Work out the finished part from the listing and answer in its coordinate system (mm). A direction names the side the tool comes from. Give positions to 0.01 mm unless a question says otherwise; leave off trailing zeros. Loops run counter-clockwise (first coordinate to the right, second up) from the corner with the lowest first, then second, coordinate; pieces in that order, holes last. Notation, with made-up numbers: (14, 46) - (19, 46) arc R12 ccw to (19, 61) - close; hole circle Ø7 at (-15.5, -2.5). An arc over 180 degrees is marked (long way). One line per question, with ' | ' between items.
from build123d import *

# Parameters (mm, degrees)
SKETCH1_R           = 4.3
SKETCH1_R_2         = 5.3
BOSS_EXTRUDE1_DEPTH = 3.3
SKETCH2_R           = 5.5
CUT_EXTRUDE1_DEPTH  = 93.907965213
FILLET1_R           = 2
SKETCH3_R           = 1.6
CUT_EXTRUDE2_DEPTH  = 93.907965213


with BuildPart() as part:
    # Sketch1 → Boss-Extrude1 (new body)
    with BuildSketch(Plane.ZY.offset(39)):
        with BuildLine():
            Line((61, 0), (21, 0))
            Line((21, 0), (21, 15))
            Line((21, 15), (-8.024613022, 54.032958367))
            ThreePointArc((-8.024613022, 54.032958367), (-8.535456817, 65.210180123), (1.639344262, 69.864712383))
            Line((1.639344262, 69.864712383), (61, 60))
            Line((61, 60), (61, 0))
        make_face()
        with Locations((20.609637027, 52.303061543)):
            Circle(SKETCH1_R, mode=Mode.SUBTRACT)
        with Locations((0, 60)):
            Circle(SKETCH1_R_2, mode=Mode.SUBTRACT)
    extrude(amount=BOSS_EXTRUDE1_DEPTH)

    # Sketch2 → Cut-Extrude1 (cut, through all)
    with BuildSketch(Plane.ZY.offset(42.3)):
        with Locations((39.931128277, 65.523132673)):
            Circle(SKETCH2_R)
    extrude(amount=-CUT_EXTRUDE1_DEPTH, mode=Mode.SUBTRACT)

    # Fillet1
    fillet1_edges = [part.edges().sort_by_distance(p)[0] for p in [
        (-40.65, 62.71535211, 44.660437774),
        (-40.65, 64.395883156, 34.547884968),
    ]]
    fillet(fillet1_edges, radius=FILLET1_R)

    # Sketch3 → Cut-Extrude2 (cut, through all)
    with BuildSketch(Plane(origin=(-39, 0, 0), x_dir=(0, 0, -1), z_dir=(1, 0, 0))):
        with Locations((-53.5, 44)):
            Circle(SKETCH3_R)
        with Locations((-39.5, 16)):
            Circle(SKETCH3_R)
        with Locations((-53.5, 16)):
            Circle(SKETCH3_R)
    extrude(amount=-CUT_EXTRUDE2_DEPTH, mode=Mode.SUBTRACT)


solid = part.part
1. Find section A-A on z = -1.5. Write down the section's boundary in (x, y), then the cut area to 3 significant figures.
Evaluation:
outline: (-42.3, 45.26) - (-39, 45.26) - (-39, 54.92) - (-42.3, 54.92) - close; (-42.3, 65.08) - (-39, 65.08) - (-39, 69.89) - (-42.3, 69.89) - close | area: 47.7 mm2
2. Find section C-C on y = 16. Write down the section's boundary in (x, z).
Evaluation:
outline: (-42.3, 20.26) - (-39, 20.26) - (-39, 37.9) - (-42.3, 37.9) - close; (-42.3, 41.1) - (-39, 41.1) - (-39, 51.9) - (-42.3, 51.9) - close; (-42.3, 55.1) - (-39, 55.1) - (-39, 61) - (-42.3, 61) - close
3. Find section D-D on z = 53.5. Write down the section's boundary in (x, y), then the cut area to 3 significant figures.
Evaluation:
outline: (-42.3, 0) - (-39, 0) - (-39, 14.4) - (-42.3, 14.4) - close; (-42.3, 17.6) - (-39, 17.6) - (-39, 42.4) - (-42.3, 42.4) - close; (-42.3, 45.6) - (-39, 45.6) - (-39, 61.25) - (-42.3, 61.25) - close | area: 181 mm2
4. Find section B-B on x = -39.8. Write down the section's boundary in (y, z) (3 decimals), then the cut area to 3 significant figures.
Evaluation:
outline: (0, 21) - (15, 21) - (54.033, -8.025) arc R10 ccw to (69.865, 1.639) - (64.596, 33.342) arc R2 ccw to (63.397, 34.859) arc R5.5 cw to (61.87, 44.043) arc R2 ccw to (62.515, 45.866) - (60, 61) - (0, 61) - close; hole circle Ø3.2 at (16, 39.5); hole circle Ø3.2 at (16, 53.5); hole circle Ø3.2 at (44, 53.5); hole circle Ø8.6 at (52.303, 20.61); hole circle Ø10.6 at (60, 0) | area: 3,340 mm2
5. Consider L1, parallel to Y at x = -40.2, z = 39.5; L2, parallel to Y at x = -41.4, z = 53.5; L3, parallel to Y at x = -40.9, z = 54. Determine where each line is inside the solid, lowest interval first.
Evaluation:
L1: 0 to 14.4, 17.6 to 60.04 | L2: 0 to 14.4, 17.6 to 42.4, 45.6 to 61.25 | L3: 0 to 14.48, 17.52 to 42.48, 45.52 to 61.16
6. Determine the mould class of faces 1 (the flat face through (-40.627, 67.267, 17.269)), 2 (the flat face through (-40.627, 34.243, 6.691)), 3 (the cylindrical face through (-40.67, 60.11, 38.95)) for opening direction Z: +Z half, -Z half, draft (parallel to the pull), parting line (faces both ways), or undercut.
Evaluation:
face 1: +Z half | face 2: -Z half | face 3: undercut
7. Flat-ended cylindrical pins translate along their axes: pin 1 (12 mm diameter, centred on y = 57, z = 4, fed in from +X); pin 2 (1 mm diameter, centred on x = -41.5, y = 5.5, fed in from -Z). Find the tip coordinate at first contact, or state that the pin passes through.
Evaluation:
pin 1: x = -39 | pin 2: z = 21
8. Which of the six approach directions +Z, -Z, +X, -X, +Y, -Y give full straight-line access (tool end or side, diameter ignored) to faces 4 (the flat face through (-41, 7, 21)), 5 (the flat face through (-42.3, 35, 34))?
Evaluation:
face 4: -Z, +X, -X, -Y | face 5: +Z, -Z, -X, +Y, -Y
